Answer from the drawing. Dimensions are ordinates in mm from the lowest x, y and z of the part. A direction names the side the tool comes from. Round coordinates to 2 decimals unless told otherwise and drop trailing zeros. Loops run counter-clockwise (first coordinate to the right, second up) from the corner with the lowest first, then second, coordinate; pieces in that order, holes last.
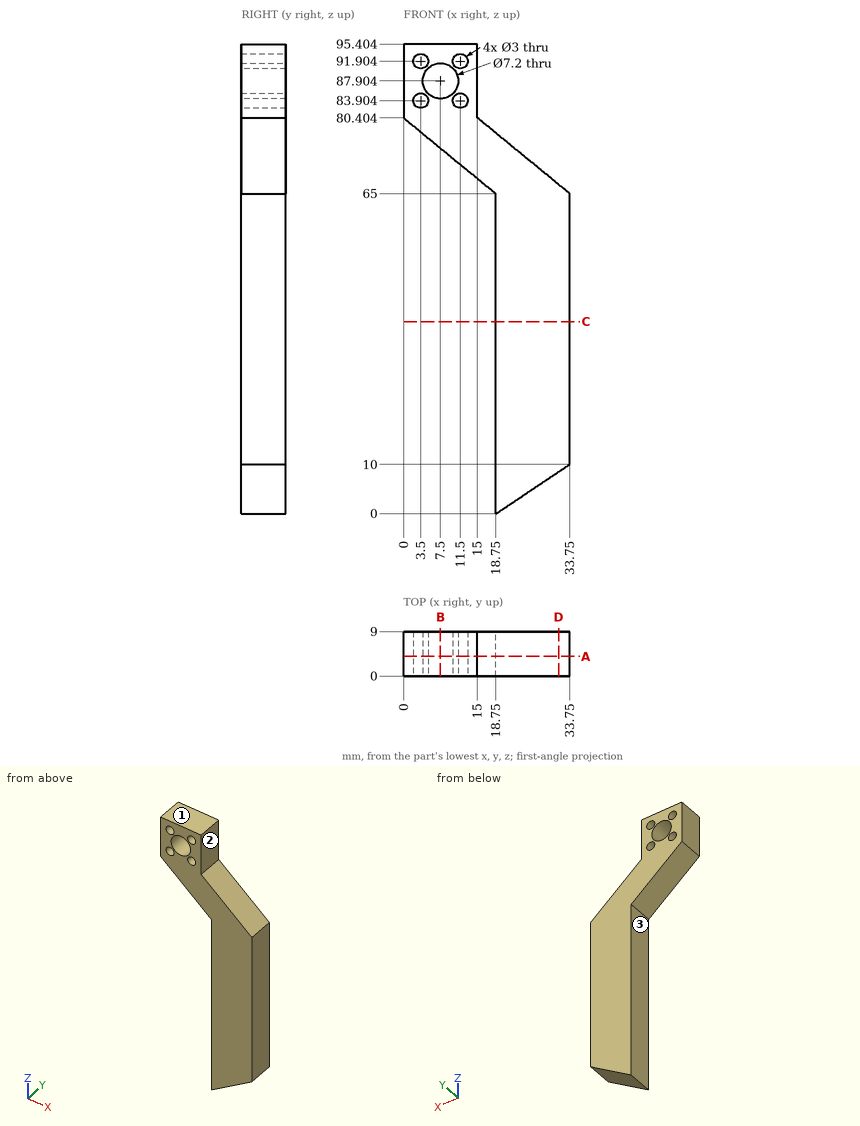
Item 1: Section C-C, the plane z = 39 is taken. Give the vertices of the cut face in (x, y), plus the area to 3 significant figures.
Item 2: For the marked faces 1, 2 and 3, determine the directions among +Z, -Z, +X, -X, +Y, -Y from which every point of the face is accessible in a straight line to the end or side of a thin tool.
Item 3: Section D-D, the plane x = 31.5 is taken. Give the vertices of the cut face in (y, z), plus the area to 3 significant figures.
Item 4: Each of these flat-tipped pins is pushed along its axis until it touches: P1, Ø3, axis at x = 29, y = 5.5, coming from the -Z side; P2, Ø2, axis at y = 5, z = 74, coming from the -X side; P3, Ø3, axis at y = 3, z = 27, coming from the -X side. Where does it stop, or does it pass through?
Item 5: Straight lines are drawn through the part: line 1 (X direction, y = 4, z = 83); line 2 (X direction, y = 7.5, z = 12); line 3 (Z direction, x = 9, y = 5) (1 decimal). For each, find the intervals that lie inside material, in ascending order.
Item 6: Section A-A, the plane y = 4 is taken. Give the vertices of the cut face in (x, z), plus the area to 3 significant figures.
Item 7: Section B-B, the plane x = 7.5 is taken. Give the vertices of the cut face in (y, z), plus the area to 3 significant figures.
Answer below:
1. outline: (18.75, 0) - (33.75, 0) - (33.75, 9) - (18.75, 9) - close
1. area: 135 mm2
2. face 1: +Z, +X, -X, +Y, -Y
2. face 2: +Z, +X, +Y, -Y
2. face 3: -Z, -X, +Y, -Y
3. outline: (0, 8.5) - (9, 8.5) - (9, 66.85) - (0, 66.85) - close
3. area: 525 mm2
4. P1: stops at z = 5.83
4. P2: stops at x = 6.58
4. P3: stops at x = 18.75
5. line 1: x = 0 to 2.3, 4.7 to 10.3, 12.7 to 15
5. line 2: x = 18.75 to 33.75
5. line 3: z = 73 to 84.6, 91.2 to 95.4
6. outline: (0, 80.4) - (18.75, 65) - (18.75, 0) - (33.75, 10) - (33.75, 65) - (15, 80.4) - (15, 95.4) - (0, 95.4) - close; hole circle Ø3 at (3.5, 83.9); hole circle Ø3 at (3.5, 91.9); hole circle Ø7.2 at (7.5, 87.9); hole circle Ø3 at (11.5, 83.9); hole circle Ø3 at (11.5, 91.9)
6. area: 1,290 mm2
7. outline: (0, 74.24) - (9, 74.24) - (9, 84.3) - (0, 84.3) - close; (0, 91.5) - (9, 91.5) - (9, 95.4) - (0, 95.4) - close
7. area: 126 mm2
